CAD build for the part. Positions are in the model's coordinates, mm. Face numbers are marked on the shaded views. A direction names the side the tool comes from. Round coordinates to 2 decimals unless told otherwise and drop trailing zeros. Order: outer loops, then holes, each group sorted by start corner. A loop starts at its lowest first (then second) coordinate and runs counter-clockwise, first axis right, second up. Notation, with made-up numbers: M 79.25,-12.5 L 124.25,-12.5 A28 cw 124.25,15.5 Z; hole C 44,23 d8. An arc over 180 degrees is marked long. Answer as a JSON object with one key per item and string values. Group by question number.
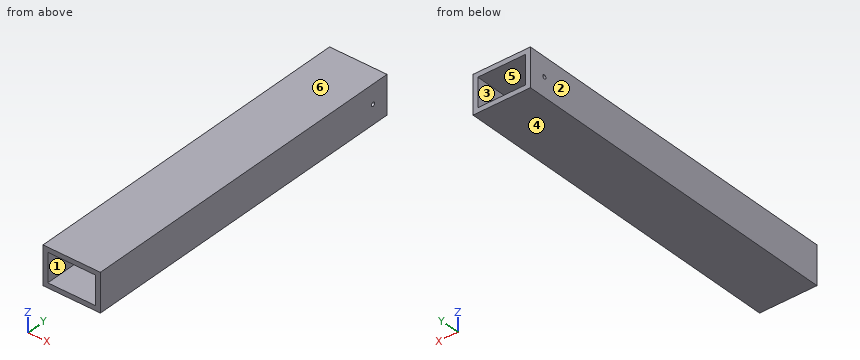
```python
from build123d import *

# Parameters (mm, degrees)
SKETCH1_W               = 76.2
SKETCH1_H               = 50.8
SKETCH1_W_2             = 63.5
SKETCH1_H_2             = 38.1
BOSS_EXTRUDE1_DEPTH     = 457.2
F_1_4_20_TAPPED_HOLE1_D = 5.1054


with BuildPart() as part:
    # Sketch1 → Boss-Extrude1 (new body)
    with BuildSketch(Plane(origin=(0, 0, 0), x_dir=(1, 0, 0), z_dir=(0, 1, 0))):
        Rectangle(SKETCH1_W, SKETCH1_H)
        Rectangle(SKETCH1_W_2, SKETCH1_H_2, mode=Mode.SUBTRACT)
    extrude(amount=BOSS_EXTRUDE1_DEPTH)

    # 1/4-20 Tapped Hole1 (through all)
    with Locations(Plane.ZY.offset(38.1)):
        with Locations((0, 434.975)):
            Hole(F_1_4_20_TAPPED_HOLE1_D / 2)


solid = part.part
```
Item 1: Cut at C-C, the plane y = 28.5. Give the cut face in (x, z).
Item 2: Cut at B-B, the plane x = -2.5. Give the cut face in (y, z).
Item 3: Two-plate mould, pull along X, no slides. Class the marked faces 1, 2, 3 and 4: +X half, -X half, draft (parallel to the pull), parting line (faces both ways), or undercut.
Item 4: 3-axis set-ups, long thin cutter, end or side, ignore diameter. For the marked faces 5 and 6: which of +Z, -Z, +X, -X, +Y, -Y reach the whole face in a straight line?
Item 5: Drill centre lines: line 1 (Y direction, x = -34.5, z = 0); line 2 (X direction, y = 373.5, z = 16.5); line 3 (Z direction, x = 16, y = 288). Where is each one in solid material? Low to high. Write a range as [from, to].
Item 6: Cut at A-A, the plane z = -9. Give the cut face in (x, y).
Response values:
{
 "1": {"outline": "M -38.1,-25.4 L 38.1,-25.4 L 38.1,25.4 L -38.1,25.4 Z; hole M -31.75,-19.05 L 31.75,-19.05 L 31.75,19.05 L -31.75,19.05 Z"},
 "2": {"outline": "M 0,-25.4 L 457.2,-25.4 L 457.2,-19.05 L 0,-19.05 Z; M 0,19.05 L 457.2,19.05 L 457.2,25.4 L 0,25.4 Z"},
 "3": {"face 1": "undercut", "face 2": "-X half", "face 3": "undercut", "face 4": "draft"},
 "4": {"face 5": "+Y, -Y", "face 6": "+Z, +X, -X, +Y, -Y"},
 "5": {"line 1": "[0, 432.42], [437.53, 457.2]", "line 2": "[-38.1, -31.75], [31.75, 38.1]", "line 3": "[-25.4, -19.05], [19.05, 25.4]"},
 "6": {"outline": "M -38.1,0 L -31.75,0 L -31.75,457.2 L -38.1,457.2 Z; M 31.75,0 L 38.1,0 L 38.1,457.2 L 31.75,457.2 Z"}
}
